from build123d import *

# Parameters (mm, degrees)
SKETCH1_R           = 15
SKETCH1_R_2         = 6
BOSS_EXTRUDE1_DEPTH = 250
CUT_EXTRUDE1_DEPTH  = 12


with BuildPart() as part:
    # Sketch1 → Boss-Extrude1 (new, symmetric)
    with BuildSketch(Plane(origin=(0, 0, 0), x_dir=(1, 0, 0), z_dir=(0, 1, 0))):
        with Locations(Location((0, 0, 0), (0, 0, 270))):
            Circle(SKETCH1_R)
        with Locations(Location((0, 0, 0), (0, 0, 270))):
            Circle(SKETCH1_R_2, mode=Mode.SUBTRACT)
    extrude(amount=BOSS_EXTRUDE1_DEPTH, both=True)

    # Sketch2 → Cut-Extrude1 (cut)
    with BuildSketch(Plane.XY):
        with BuildLine():
            Line((-6, 200), (-6, 174.999998924))
            ThreePointArc((-6, 174.999998924), (0, 168.999998924), (6, 174.999998924))
            Line((6, 174.999998924), (6, 200))
            ThreePointArc((6, 200), (0, 206), (-6, 200))
        make_face()
    extrude(amount=-CUT_EXTRUDE1_DEPTH, mode=Mode.SUBTRACT)


solid = part.part
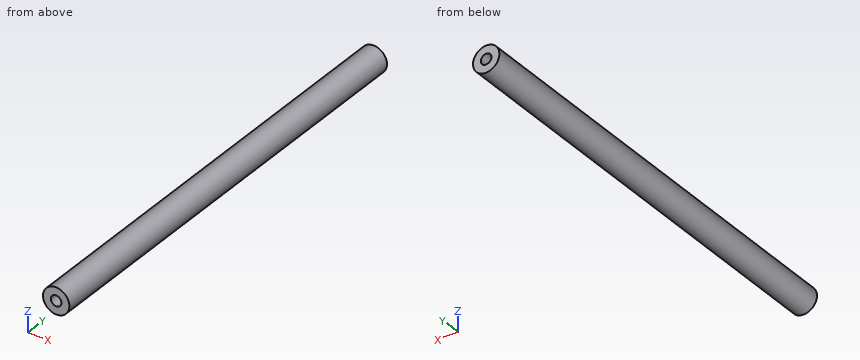
Check sheet for the modelled part. Datum: model origin and axes. Units: mm. Give positions to 0.01 mm unless a question says otherwise; leave off trailing zeros. Loops run counter-clockwise (first coordinate to the right, second up) from the corner with the lowest first, then second, coordinate; pieces in that order, holes last. Notation, with made-up numbers: M 74,42 L 119,42 A23 cw 119,68 Z; hole C -31.75,17.5 d10. An arc over 180 degrees is marked long. Return JSON: item names as keys, results as strings. Group by question number.
1. Cross-section at A-A on x = 0. Record the boundary of the cut face in (y, z), plus the area to 3 significant figures.
2. Thickness scan on L1, parallel to X at y = -117, z = 1; L2, parallel to X at y = 87.5, z = 0; L3, parallel to Y at x = -3.75, z = -6. Record the ranges inside material, lowest first.
3. Go/stop test with flat-tipped pins: pin 1 (3 mm diameter, centred on x = -11.5, y = -179.5, fed in from -Z); pin 2 (6 mm diameter, centred on y = 186.5, z = -4.5, fed in from +X); pin 3 (1 mm diameter, centred on x = -3.5, z = 3, fed in from -Y); pin 4 (9.5 mm diameter, centred on y = 185.5, z = -7, fed in from -X). Record where each tip stops, or that it passes through.
4. Cross-section at B-B on y = -9. Record the boundary of the cut face in (x, z), plus the area to 3 significant figures.
Return value:
{
 "1": {"outline": "M -250,-15 L 250,-15 L 250,-6 L 206,-6 L 206,-12 L 169,-12 L 169,-6 L -250,-6 Z; M -250,6 L 250,6 L 250,15 L -250,15 Z", "area": "8,780 mm^2"},
 "2": {"L1": "-14.97 to -5.92, 5.92 to 14.97", "L2": "-15 to -6, 6 to 15", "L3": "-250 to 170.32, 204.68 to 250"},
 "3": {"pin 1": "z = -11.18", "pin 2": "x = 14.92", "pin 3": "through", "pin 4": "x = -14.83"},
 "4": {"outline": "C 0,0 d30; hole C 0,0 d12", "area": "594 mm^2"}
}
